Could you check a few things on this model? Use its own coordinates, in mm. Face numbers are marked on the shaded views. A direction names the side the tool comes from. Coordinates: 2 decimals unless noted, no trailing zeros. Write each loop counter-clockwise with the first axis right and the second up, starting at its lowest first coordinate (ties: lowest second). Pieces come first, ordered by that corner, then holes. Notation, with made-up numbers: (77, 76.5) - (90, 76.5) arc R30 ccw to (90, 111.5) - close; hole circle Ø11 at (77, 2). An arc over 180 degrees is marked (long way). Answer as a JSON object with one key per item and string values. Group by question number.
1) Please list where these lines run through material, in increasing order: line 1 along Z through (x, y) = (-69, 6); line 2 along Z through (x, y) = (-28, 33); line 3 along X through (y, z) = (3.5, 0.9).
2) If we section it at B-B (y = 26.5): Write out the boundary of the cut face in (x, z).
3) On a 3-axis mill with a long thin cutter (end or side, diameter ignored), from which of +Z, -Z, +X, -X, +Y, -Y can I reach the whole of each face in a straight line? I mean the marked faces 1 and 2. Say none if no direction works.
4) If we section it at A-A (x = -28): Write out the boundary of the cut face in (y, z).
5) Will these pins go through, and if not, where does the flat tip stop? pin 1 Ø2 at (x, y) = (3.5, 0.5) entering from -Z; pin 2 Ø2 at (y, z) = (22, 1) entering from -X; pin 3 Ø1.6 at (y, z) = (21.5, 1) entering from +X.
```python
from build123d import *

# Parameters (mm, degrees)
F2_DEPTH = 140
F3_DEPTH = 145
F4_DEPTH = 5


with BuildPart() as f2:
    # F0 (on Right) → F2 (new body)
    with BuildSketch(Plane.YZ):
        with BuildLine():
            ThreePointArc((0, 1), (0.292893, 0.292893), (1, 0))
            Line((1, 0), (31, 0))
            ThreePointArc((31, 0), (31.707107, 0.292893), (32, 1))
            Line((32, 1), (35, 1))
            Line((35, 1), (35, 2))
            Line((35, 2), (0, 2))
            Line((0, 2), (0, 1))
        make_face()
    extrude(amount=-F2_DEPTH)

    # F1 (on Right) → F3 (join)
    with BuildSketch(Plane.YZ):
        with BuildLine():
            Line((0, 3), (0, 2))
            Line((0, 2), (2, 2))
            Line((2, 2), (2, 3))
            ThreePointArc((2, 3), (1.707107, 3.707107), (1, 4))
            ThreePointArc((1, 4), (0.292893, 3.707107), (0, 3))
        make_face()
    extrude(amount=-F3_DEPTH)

    # F1 (on Right) → F4 (join)
    with BuildSketch(Plane.YZ):
        with BuildLine():
            Line((0, 3), (0, 2))
            Line((0, 2), (2, 2))
            Line((2, 2), (2, 3))
            ThreePointArc((2, 3), (1.707107, 3.707107), (1, 4))
            ThreePointArc((1, 4), (0.292893, 3.707107), (0, 3))
        make_face()
    extrude(amount=F4_DEPTH)


solid = f2.part
```
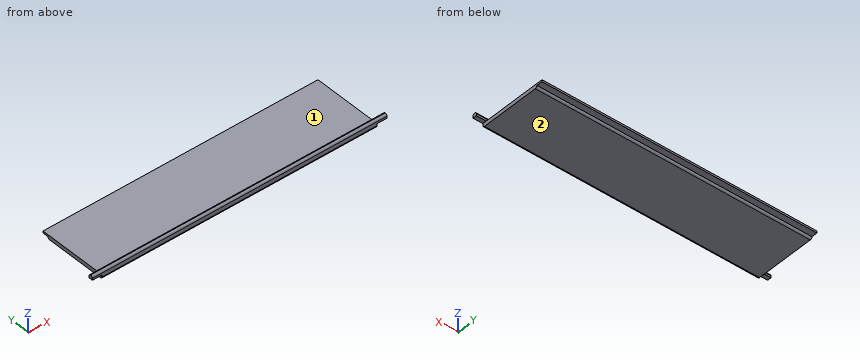
Here are the results:
{
 "1": {"line 1": "z = 0 to 2", "line 2": "z = 1 to 2", "line 3": "x = -140 to 0"},
 "2": {"outline": "(-140, 0) - (0, 0) - (0, 2) - (-140, 2) - close"},
 "3": {"face 1": "+Z, +X, -X, +Y", "face 2": "-Z, +X, -X, +Y, -Y"},
 "4": {"outline": "(0, 1) arc R1 ccw to (1, 0) - (31, 0) arc R1 ccw to (32, 1) - (35, 1) - (35, 2) - (2, 2) - (2, 3) arc R1 ccw to (1, 4) arc R1 ccw to (0, 3) - close"},
 "5": {"pin 1": "stops at z = 2", "pin 2": "stops at x = -140", "pin 3": "stops at x = 0"}
}
